from build123d import *

# Parameters (mm, degrees)
SKETCH1_W           = 176
SKETCH1_H           = 10
BOSS_EXTRUDE1_DEPTH = 10
SKETCH2_W           = 12
SKETCH2_H           = 10
BOSS_EXTRUDE2_DEPTH = 50
SKETCH3_W           = 10
SKETCH3_H           = 10
SKETCH3_W_2         = 12
BOSS_EXTRUDE3_DEPTH = 23
SKETCH4_W           = 12
SKETCH4_H           = 10
BOSS_EXTRUDE4_DEPTH = 115
SKETCH6_W           = 4
SKETCH6_H           = 4
CUT_EXTRUDE1_DEPTH  = 5
SKETCH7_W           = 4
SKETCH7_H           = 4
CUT_EXTRUDE2_DEPTH  = 5


with BuildPart() as part:
    # Sketch1 → Boss-Extrude1 (new body)
    with BuildSketch(Plane.XY):
        with Locations((88, 5)):
            Rectangle(SKETCH1_W, SKETCH1_H)
    extrude(amount=BOSS_EXTRUDE1_DEPTH)

    # Sketch2 → Boss-Extrude2 (add)
    with BuildSketch(Plane(origin=(0, 0, 0), x_dir=(-1, 0, 0), z_dir=(0, 0, -1))):
        with Locations((-87.845258849, 5)):
            Rectangle(SKETCH2_W, SKETCH2_H)
    extrude(amount=BOSS_EXTRUDE2_DEPTH)

    # Sketch3 → Boss-Extrude3 (add)
    with BuildSketch(Plane(origin=(0, 0, 0), x_dir=(-1, 0, 0), z_dir=(0, 0, -1))):
        with Locations((-5, 5)):
            Rectangle(SKETCH3_W, SKETCH3_H)
        with Locations((-170, 5)):
            Rectangle(SKETCH3_W_2, SKETCH3_H)
    extrude(amount=BOSS_EXTRUDE3_DEPTH)

    # Mirror6: part across plane


with BuildPart() as part_1:
    add(part.part)
    add(part.part.mirror(Plane.XY.offset(-50)))

    # Sketch4 → Boss-Extrude4 (add)
    with BuildSketch(Plane.XZ):
        with Locations((87.845258849, 5)):
            Rectangle(SKETCH4_W, SKETCH4_H)
        with Locations((87.845258849, -105)):
            Rectangle(SKETCH4_W, SKETCH4_H)
    extrude(amount=BOSS_EXTRUDE4_DEPTH)

    # Sketch6 → Cut-Extrude1 (cut)
    with BuildSketch(Plane.XY.offset(10)):
        with Locations((87.80305242, -110.022825142)):
            Rectangle(SKETCH6_W, SKETCH6_H)
    extrude(amount=-CUT_EXTRUDE1_DEPTH, mode=Mode.SUBTRACT)

    # Sketch7 → Cut-Extrude2 (cut)
    with BuildSketch(Plane(origin=(0, 0, -110), x_dir=(-1, 0, 0), z_dir=(0, 0, -1))):
        with Locations((-87.845258849, -110)):
            Rectangle(SKETCH7_W, SKETCH7_H)
    extrude(amount=-CUT_EXTRUDE2_DEPTH, mode=Mode.SUBTRACT)


solid = part_1.part
The model under review builds one solid part; all positions refer to its coordinate system, in mm. A direction names the side the tool comes from. Round coordinates to 2 decimals unless told otherwise and drop trailing zeros. Loops run counter-clockwise (first coordinate to the right, second up) from the corner with the lowest first, then second, coordinate; pieces in that order, holes last. Notation, with made-up numbers: M 78.25,-14.75 L 105.25,-14.75 A4 ccw 105.25,-10.75 Z; hole C 7.25,-1 d2. An arc over 180 degrees is marked long. Answer as CSV lines item,"result".
1. We need section C-C (x = 104). Give the boundary of the cut face in (y, z), plus the area to 3 significant figures.
Outcome:
outline,"M 0,-110 L 10,-110 L 10,-100 L 0,-100 Z; M 0,0 L 10,0 L 10,10 L 0,10 Z"
area,"200 mm2"
2. We need section A-A (y = -32). Give the boundary of the cut face in (x, z), plus the area to 3 significant figures.
Outcome:
outline,"M 81.85,-110 L 93.85,-110 L 93.85,-100 L 81.85,-100 Z; M 81.85,0 L 93.85,0 L 93.85,10 L 81.85,10 Z"
area,"240 mm2"
3. Draft analysis for pull direction Y (two halves, no side actions). For faces 1 (the face through (45, 5, -100)), 2 (the face through (88, -108, -108)), 3 (the face through (88, -115, 5)), state which applies: pulls with the +Y half, pulls with the -Y half, needs draft (parallel to the pull), parting line crosses it, or undercut.
Outcome:
face 1,"needs draft"
face 2,"undercut"
face 3,"pulls with the -Y half"
4. To check wall thickness, follow L1, parallel to Z at x = 82, y = -108.5; L2, parallel to Y at x = 93.5, z = -26.5; L3, parallel to X at y = -102, z = 5.5. State the ranges of each line that lie inside material, in increasing order. Write a range as [from, to].
Outcome:
L1,"z = [-110, -100], [0, 10]"
L2,"y = [0, 10]"
L3,"x = [81.85, 93.85]"
5. For faces 4 (the face through (145, 0, -101)), 5 (the face through (88, -110, -105)), 6 (the face through (164, 5, -89)), 7 (the face through (88, -57, 0)), list the 3-axis set-ups (+Z, -Z, +X, -X, +Y, -Y) from which the entire face can be reached by the end or side of a thin tool; tool diameter is ignored.
Outcome:
face 4,"+Z, -Z, +X, -Y"
face 5,"-Z"
face 6,"+Y, -Y"
face 7,"+X, -X, -Y"
6. We need section D-D (z = -41.5). Give the boundary of the cut face in (x, y), plus the area to 3 significant figures.
Outcome:
outline,"M 81.85,0 L 93.85,0 L 93.85,10 L 81.85,10 Z"
area,"120 mm2"
7. We need section B-B (z = -96). Give the boundary of the cut face in (x, y).
Outcome:
outline,"M 0,0 L 10,0 L 10,10 L 0,10 Z; M 81.85,0 L 93.85,0 L 93.85,10 L 81.85,10 Z; M 164,0 L 176,0 L 176,10 L 164,10 Z"
8. Insertion check: pin 1 Ø1.2 at (y, z) = (-109, -108) entering from +X; pin 2 Ø4.5 at (y, z) = (-110, 8) entering from -X; pin 3 Ø13 at (x, z) = (90, -46) entering from -Y; pin 4 Ø11 at (y, z) = (3, -16) entering from -X. Each pin has a flat end and moves straight along its axis. Give the tip position at first contact, or say it passes through.
Outcome:
pin 1,"stops at x = 93.85"
pin 2,"stops at x = 81.85"
pin 3,"stops at y = 0"
pin 4,"stops at x = 0"
